```python
from build123d import *

# Parameters (mm, degrees)
SKETCH1_W           = 30
SKETCH1_H           = 50
BOSS_EXTRUDE1_DEPTH = 3
SKETCH2_W           = 30
SKETCH2_H           = 5
BOSS_EXTRUDE2_DEPTH = 25
FILLET1_R           = 3


with BuildPart() as part:
    # Sketch1 → Boss-Extrude1 (new body)
    with BuildSketch(Plane.XY):
        Rectangle(SKETCH1_W, SKETCH1_H)
        with BuildLine():
            Line((-11.85, 8), (-11.85, 16))
            ThreePointArc((-11.85, 16), (-10, 17.85), (-8.15, 16))
            Line((-8.15, 16), (-8.15, 8))
            ThreePointArc((-8.15, 8), (-10, 6.15), (-11.85, 8))
        make_face(mode=Mode.SUBTRACT)
        with BuildLine():
            Line((11.85, 8), (11.85, 16))
            ThreePointArc((11.85, 16), (10, 17.85), (8.15, 16))
            Line((8.15, 16), (8.15, 8))
            ThreePointArc((8.15, 8), (10, 6.15), (11.85, 8))
        make_face(mode=Mode.SUBTRACT)
        with BuildLine():
            Line((11.835217348, 1.894233852), (11.796480023, -6.105672361))
            ThreePointArc((11.796480023, -6.105672361), (9.937543705, -7.946692666), (8.0965234, -6.087756348))
            Line((8.0965234, -6.087756348), (8.135260724, 1.912149865))
            ThreePointArc((8.135260724, 1.912149865), (9.994197043, 3.75317017), (11.835217348, 1.894233852))
        make_face(mode=Mode.SUBTRACT)
        with BuildLine():
            Line((-11.864504809, 2.008993176), (-11.903242133, -5.990913037))
            ThreePointArc((-11.903242133, -5.990913037), (-10.062221828, -7.849849355), (-8.203285509, -6.008829049))
            Line((-8.203285509, -6.008829049), (-8.164548185, 1.991077164))
            ThreePointArc((-8.164548185, 1.991077164), (-10.00556849, 3.850013482), (-11.864504809, 2.008993176))
        make_face(mode=Mode.SUBTRACT)
    extrude(amount=BOSS_EXTRUDE1_DEPTH)

    # Sketch2 → Boss-Extrude2 (add)
    with BuildSketch(Plane.XY):
        with Locations((0, -27.5)):
            Rectangle(SKETCH2_W, SKETCH2_H)
    extrude(amount=BOSS_EXTRUDE2_DEPTH)

    # Fillet1
    fillet1_edges = [part.edges().sort_by_distance(p)[0] for p in [
        (0, -30, 25),
        (0, -30, 0),
        (0, -25, 3),
        (0, 25, 0),
    ]]
    fillet(fillet1_edges, radius=FILLET1_R - 0.0001)  # a hair under: the kernel refuses the full size


solid = part.part
```
Check sheet for the modelled part. Datum: model origin and axes. Units: mm. A direction names the side the tool comes from. Round coordinates to 2 decimals unless told otherwise and drop trailing zeros. Loops run counter-clockwise (first coordinate to the right, second up) from the corner with the lowest first, then second, coordinate; pieces in that order, holes last. Notation, with made-up numbers: (-9.5, -6) -> (29.5, -6) arc R8 ccw to (29.5, 3) -> close; hole circle Ø4 at (51, 62). An arc over 180 degrees is marked (long way). Answer in a Markdown table with one row per item.
Q1. Release check for a two-part mould opening along X. For faces 1 (the face through (-9.96, 3.85, 1.48)), 2 (the face through (-15, -17, 2)), 3 (the face through (0, -26, 25)) record: released by +X, released by -X, zero draft, split by the parting line, or undercut.
Data:
| item | result |
|---|---|
| face 1 | undercut |
| face 2 | released by -X |
| face 3 | zero draft |
Q2. Thickness scan on L1, parallel to Z at x = -5, y = -21.5; L2, parallel to Z at x = -9.5, y = -24; L3, parallel to Y at x = 6.75, z = 10.25. Record the ranges inside material, lowest first.
Data:
| item | result |
|---|---|
| L1 | z = 0 to 3 |
| L2 | z = 0 to 3.76 |
| L3 | y = -30 to -25 |
Q3. Sectioned sample at A-A on x = 9.25. Give the number of separate pieces and of enclosed holes in the cut face, then the cut area to 3 significant figures.
Data:
| item | result |
|---|---|
| separate pieces | 3 |
| enclosed holes | 0 |
| area | 203 mm^2 |
Q4. Go/stop test with flat-tipped pins: P1, Ø15, axis at x = -2, z = 11.5, coming from the +Y side; P2, Ø6, axis at x = -9.5, z = 13, coming from the +Y side; P3, Ø8, axis at y = -17.5, z = 13.5, coming from the -X side. Record where each tip stops, or that it passes through.
Data:
| item | result |
|---|---|
| P1 | stops at y = -24.24 |
| P2 | stops at y = -25 |
| P3 | passes through |
Q5. Sectioned sample at B-B on y = 17. Enter the section's corners in (x, z), then the cut area to 3 significant figures.
Data:
| item | result |
|---|---|
| outline | (-15, 0) -> (-11.56, 0) -> (-11.56, 3) -> (-15, 3) -> close; (-8.44, 0) -> (8.44, 0) -> (8.44, 3) -> (-8.44, 3) -> close; (11.56, 0) -> (15, 0) -> (15, 3) -> (11.56, 3) -> close |
| area | 71.3 mm^2 |
Q6. Set-up check for faces 4 (the face through (9.954, 3.753, 1.479)), 5 (the face through (0, -30, 12)), 6 (the face through (0, 2, 3)): record each of +Z, -Z, +X, -X, +Y, -Y from which the full face is reachable in a straight line by a thin tool's end or side.
Data:
| item | result |
|---|---|
| face 4 | +Z, -Z |
| face 5 | +Z, -Z, +X, -X, -Y |
| face 6 | +Z, +X, -X, +Y |
Q7. Sectioned sample at D-D on z = 11.25. Enter the section's corners in (x, y).
Data:
| item | result |
|---|---|
| outline | (-15, -30) -> (15, -30) -> (15, -25) -> (-15, -25) -> close |
